from build123d import *

# Parameters (mm, degrees)
BASE_FLANGE1_DEPTH              = 2.7
EDGE_FLANGE1_STRIP_W            = 14.8
EDGE_FLANGE1_STRIP_H            = 2.7
EDGE_FLANGE1_STRIP_CUT_DEPTH    = 91.7
EDGE_FLANGE1_RELIEF_W           = 20.2
EDGE_FLANGE1_RELIEF_H           = 5.4
EDGE_FLANGE1_RELIEF_CUT_DEPTH   = 2.7
EDGE_FLANGE1_STRIP_2_W          = 14.8
EDGE_FLANGE1_STRIP_2_H          = 2.7
EDGE_FLANGE1_STRIP_CUT_2_DEPTH  = 528.3
EDGE_FLANGE1_RELIEF_2_W         = 20.2
EDGE_FLANGE1_RELIEF_2_H         = 5.4
EDGE_FLANGE1_RELIEF_CUT_2_DEPTH = 2.7
EDGE_FLANGE1_DEPTH              = 91.7
EDGE_FLANGE1_BEND_DEPTH         = 528.3


# Sheet-metal steps are written as plain solids
with BuildPart() as part:
    # Sketch1 → Base-Flange1 (new body)
    with BuildSketch(Plane.XY):
        Polygon((43, 700), (0, 700), (0, 0), (113, 0), (113, 91.7), (43, 171.7), align=None)
    extrude(amount=-BASE_FLANGE1_DEPTH)

    # Edge-Flange1 strip (across the edge) → Edge-Flange1 strip cut (cut)
    with BuildSketch(Plane(origin=(113, 91.7, -2.7), x_dir=(-1, 0, 0), z_dir=(0, -1, 0))):
        with Locations((-2.7, -1.35)):
            Rectangle(EDGE_FLANGE1_STRIP_W, EDGE_FLANGE1_STRIP_H)
    extrude(amount=EDGE_FLANGE1_STRIP_CUT_DEPTH, mode=Mode.SUBTRACT)

    # Edge-Flange1 relief (on the sheet) → Edge-Flange1 relief cut (cut)
    with BuildSketch(Plane(origin=(108.3, 91.7, -2.7), x_dir=(-1, 0, 0), z_dir=(0, 0, -1))):
        with Locations((-4.7, 2.7)):
            Rectangle(EDGE_FLANGE1_RELIEF_W, EDGE_FLANGE1_RELIEF_H)
    extrude(amount=-EDGE_FLANGE1_RELIEF_CUT_DEPTH, mode=Mode.SUBTRACT)

    # Edge-Flange1 strip 2 (across the edge) → Edge-Flange1 strip cut 2 (cut)
    with BuildSketch(Plane(origin=(43, 700, -2.7), x_dir=(-1, 0, 0), z_dir=(0, -1, 0))):
        with Locations((-2.7, -1.35)):
            Rectangle(EDGE_FLANGE1_STRIP_2_W, EDGE_FLANGE1_STRIP_2_H)
    extrude(amount=EDGE_FLANGE1_STRIP_CUT_2_DEPTH, mode=Mode.SUBTRACT)

    # Edge-Flange1 relief 2 (on the sheet) → Edge-Flange1 relief cut 2 (cut)
    with BuildSketch(Plane(origin=(38.3, 700, -2.7), x_dir=(-1, 0, 0), z_dir=(0, 0, -1))):
        with Locations((-4.7, -531)):
            Rectangle(EDGE_FLANGE1_RELIEF_2_W, EDGE_FLANGE1_RELIEF_2_H)
    extrude(amount=-EDGE_FLANGE1_RELIEF_CUT_2_DEPTH, mode=Mode.SUBTRACT)

    # Edge-Flange1 section (across the edge) → Edge-Flange1 (add)
    with BuildSketch(Plane(origin=(113, 91.7, -2.7), x_dir=(-1, 0, 0), z_dir=(0, -1, 0))):
        with BuildLine():
            Line((0, 2), (0, 47.3))
            Line((0, 47.3), (2.7, 47.3))
            Line((2.7, 47.3), (2.7, 2))
            ThreePointArc((2.7, 2), (3.285786438, 0.585786438), (4.7, 0))
            Line((4.7, 0), (4.7, -2.7))
            ThreePointArc((4.7, -2.7), (1.376598128, -1.323401872), (0, 2))
        make_face()
    extrude(amount=EDGE_FLANGE1_DEPTH)

    # Edge-Flange1 section 2 (across the edge) → Edge-Flange1 bend (add)
    with BuildSketch(Plane(origin=(43, 700, -2.7), x_dir=(-1, 0, 0), z_dir=(0, -1, 0))):
        with BuildLine():
            Line((0, 2), (0, 47.3))
            Line((0, 47.3), (2.7, 47.3))
            Line((2.7, 47.3), (2.7, 2))
            ThreePointArc((2.7, 2), (3.285786438, 0.585786438), (4.7, 0))
            Line((4.7, 0), (4.7, -2.7))
            ThreePointArc((4.7, -2.7), (1.376598128, -1.323401872), (0, 2))
        make_face()
    extrude(amount=EDGE_FLANGE1_BEND_DEPTH)


solid = part.part
Can you work these out from the model? Positions are in its coordinate system, mm. A direction names the side the tool comes from. Coordinates: 2 decimals unless noted, no trailing zeros. Loops run counter-clockwise (first coordinate to the right, second up) from the corner with the lowest first, then second, coordinate; pieces in that order, holes last. Notation, with made-up numbers: M -18.5,82.5 L 9.5,82.5 A6 ccw 9.5,88.5 Z; hole C -27,59 d8. An arc over 180 degrees is marked long. Return JSON: item names as keys, results as strings. Group by question number.
Item 1: Thinking about a two-plate mould opening in X: for faces 3 (the flat face through (113, 46, -27)), 4 (the flat face through (29, 277, -2.7)), 5 (the flat face through (110.3, 46, -28)), which applies, released by +X, released by -X, zero draft, split by the parting line, or undercut?
Item 2: Imagine slicing it at B-B (y = 371.5). Please give me the cut outline in (x, z).
Item 3: If I drill on L1, parallel to X at y = 58, z = -25.5; L2, parallel to Z at x = 28, y = 433.5; L3, parallel to X at y = 655.5, z = -11.5, over which ranges is the centre line in solid material (lowest first)? Write a range as from..to.
Item 4: Imagine slicing it at C-C (x = 81.5). Please give me the cut outline in (y, z), and give its area (3 significant figures).
Item 5: Imagine slicing it at A-A (z = -43.5). Please give me the cut outline in (x, y).
Item 6: Imagine slicing it at D-D (y = 140.5). Please give me the cut outline in (x, z), and give its area (3 significant figures).
Item 7: On a 3-axis mill with a long thin cutter (end or side, diameter ignored), from which of +Z, -Z, +X, -X, +Y, -Y can I reach the whole of each face in a straight line? I mean faces 1 (the flat face through (41, 700, -18)), 2 (the flat face through (40.3, 440, -28)). Say none if no direction works.
Item 8: I'm going to push flat-ended pins straight in: pin 1 Ø1.4 at (y, z) = (170.5, -1) entering from +X; pin 2 Ø1.5 at (x, y) = (14, 557.5) entering from -Z; pin 3 Ø11 at (x, z) = (110, -16) entering from +Y. Where does each tip first touch, or does it pass through?
Verdict:
{
 "1": {"face 3": "released by +X", "face 4": "zero draft", "face 5": "released by -X"},
 "2": {"outline": "M 0,-2.7 L 38.3,-2.7 A2 cw 40.3,-4.7 L 40.3,-50 L 43,-50 L 43,-4.7 A4.7 ccw 38.3,0 L 0,0 Z"},
 "3": {"L1": "x = 110.3..113", "L2": "z = -2.7..0", "L3": "x = 40.3..43"},
 "4": {"outline": "M 0,-2.7 L 127.7,-2.7 L 127.7,0 L 0,0 Z", "area": "345 mm^2"},
 "5": {"outline": "M 40.3,171.7 L 43,171.7 L 43,700 L 40.3,700 Z; M 110.3,0 L 113,0 L 113,91.7 L 110.3,91.7 Z"},
 "6": {"outline": "M 0,-2.7 L 70.3,-2.7 L 70.3,0 L 0,0 Z", "area": "190 mm^2"},
 "7": {"face 1": "+Z, -Z, +X, -X, +Y", "face 2": "-Z, -X, +Y, -Y"},
 "8": {"pin 1": "stops at x = 32.9", "pin 2": "stops at z = -2.7", "pin 3": "stops at y = 91.7"}
}
